Verification items for the finished model (mm, model axes). Face numbers are marked on the shaded views. A direction names the side the tool comes from. Coordinates: 2 decimals unless noted, no trailing zeros. Order: outer loops, then holes, each group sorted by start corner. A loop starts at its lowest first (then second) coordinate and runs counter-clockwise, first axis right, second up. Notation, with made-up numbers: M 36.5,59.25 L 52.5,59.25 A5 cw 52.5,66.25 Z; hole C 13.5,53 d9. An arc over 180 degrees is marked long. Answer as a JSON object with one key per item and string values. Group by question number.
(1) Material ranges on line 1 (X direction, y = -3.5, z = 15); line 2 (Z direction, x = 17, y = -8); line 3 (X direction, y = -89, z = 162), recorded low to high.
(2) Cross-section at A-A (x = 3.5). Enter the section's corners in (y, z).
(3) Access from +Z, -Z, +X, -X, +Y, -Y to the whole of each face (thin tool, end or side, straight path). Record for the marked faces 1, 2, 3, 4 and 5.
(4) Mould release check, pull along Y, two halves, no side actions. Record for the marked faces 6, 7 and 8: released by +Y, released by -Y, zero draft, split by the parting line, or undercut.
(5) Gauge pin test, flat ends, axial feed: pin 1 Ø2 at (x, z) = (-37.5, 45) entering from +Y; pin 2 Ø3 at (x, z) = (-17.5, 98) entering from +Y; pin 3 Ø5 at (x, z) = (-9.5, 44) entering from -Y. Record the tip position at first contact, or that the pin passes through.
(6) Cross-section at B-B (y = -99). Enter the section's corners in (x, z).
from build123d import *

# Parameters (mm, degrees)
ESQUISSE1_W                         = 50
ESQUISSE1_H                         = 70
ESQUISSE1_R                         = 2
ESQUISSE1_R_2                       = 20
BOSS_EXTRU_1_DEPTH                  = 10
BOSS_EXTRU_2_REACH                  = 57.317
ESQUISSE13_R                        = 21.5
ESQUISSE13_R_2                      = 20
BOSS_EXTRU_2_DIRECTION_2_DEPTH      = 90
ESQUISSE19_R                        = 21.5
ESQUISSE19_R_2                      = 20
R_VOLUTION5_ANGLE                   = 70
ESQUISSE23_R                        = 21.5
ESQUISSE23_R_2                      = 20
BOSS_EXTRU_3_DEPTH                  = 70
ESQUISSE24_W                        = 23
ESQUISSE24_H                        = 16.3
ENL_V_MAT_EXTRU_1_DEPTH             = 10
BOSS_EXTRU_4_DEPTH                  = 13
BOSS_EXTRU_4_DIRECTION_2_REACH      = 242.506
BOSS_EXTRU_4_DIRECTION_2_END_RADIUS = 21.5
ESQUISSE28_W                        = 4
ESQUISSE28_H                        = 4
BOSS_EXTRU_5_DEPTH                  = 23


with BuildPart() as part:
    # Esquisse1 → Boss.-Extru.1 (new body)
    with BuildSketch(Plane.XY):
        with Locations((-5.186655458, -0.726415094)):
            Rectangle(ESQUISSE1_W, ESQUISSE1_H)
        with Locations((-5.186655458, 25.273584906)):
            Circle(ESQUISSE1_R, mode=Mode.SUBTRACT)
        with Locations((-5.186655458, -30.726415094)):
            Circle(ESQUISSE1_R, mode=Mode.SUBTRACT)
        with Locations((-5.186655458, -0.726415094)):
            Circle(ESQUISSE1_R_2, mode=Mode.SUBTRACT)
    extrude(amount=BOSS_EXTRU_1_DEPTH)

    # Boss.-Extru.2: up to this plane
    boss_extru_2_end = Plane(origin=(0, 0, 10), z_dir=(0, 0, 1))
    # Esquisse13 → Boss.-Extru.2 (add, up to the surface)
    with BuildSketch(Plane(origin=(0, -7.393134718, 20.312470696), x_dir=(1, 0, 0), z_dir=(0, -0.34202014332566283, 0.9396926207859106)), mode=Mode.PRIVATE) as boss_extru_2_sk1:
        with Locations(Location((-5.554517745, 2.737594529, 0), (0, 0, 270))):
            Circle(ESQUISSE13_R)
        with Locations(Location((-5.554517745, 2.737594529, 0), (0, 0, 29.306498897))):
            Circle(ESQUISSE13_R_2, mode=Mode.SUBTRACT)
    boss_extru_2_tool1 = split(extrude(boss_extru_2_sk1.sketch, amount=-BOSS_EXTRU_2_REACH, mode=Mode.PRIVATE), bisect_by=boss_extru_2_end, keep=Keep.BOTH, mode=Mode.PRIVATE)
    add(boss_extru_2_tool1.solids().sort_by_distance((-5.554518, 14.811316, 28.39423))[0])

    # Esquisse13 → Boss.-Extru.2 direction 2 (add)
    with BuildSketch(Plane(origin=(0, -7.393134718, 20.312470696), x_dir=(1, 0, 0), z_dir=(0, -0.34202014332566283, 0.9396926207859106))):
        with Locations(Location((-5.554517745, 2.737594529, 0), (0, 0, 270))):
            Circle(ESQUISSE13_R)
        with Locations(Location((-5.554517745, 2.737594529, 0), (0, 0, 29.306498897))):
            Circle(ESQUISSE13_R_2, mode=Mode.SUBTRACT)
    extrude(amount=BOSS_EXTRU_2_DIRECTION_2_DEPTH)

    # Esquisse19 → Révolution5 (revolve)
    with BuildSketch(Plane(origin=(0, -38.174947617, 104.884806567), x_dir=(1, 0, 0), z_dir=(0, -0.34202014332566294, 0.9396926207859106))):
        with Locations(Location((-5.554517745, 2.737594529, 0), (0, 0, 90))):
            Circle(ESQUISSE19_R)
        with Locations(Location((-5.554517745, 2.737594529, 0), (0, 0, 90))):
            Circle(ESQUISSE19_R_2, mode=Mode.SUBTRACT)
    revolve(axis=Axis((-5.554579986, -94.784211414, 84.280719561), (1, 0, 0)), revolution_arc=R_VOLUTION5_ANGLE)

    # Esquisse23 → Boss.-Extru.3 (add)
    with BuildSketch(Plane.XZ.offset(94.784211414)):
        with Locations(Location((-5.554579986, 147.260634339, 0), (0, 0, 270))):
            Circle(ESQUISSE23_R)
        with Locations(Location((-5.554579986, 147.260634339, 0), (0, 0, 270.000178307))):
            Circle(ESQUISSE23_R_2, mode=Mode.SUBTRACT)
    extrude(amount=BOSS_EXTRU_3_DEPTH)

    # Esquisse24 → Enlèv. mat.-Extru.1 (cut)
    with BuildSketch(Plane.ZY.offset(27.186655458)):
        with Locations((46.360115203, -11.15)):
            Rectangle(ESQUISSE24_W, ESQUISSE24_H)
    extrude(amount=-ENL_V_MAT_EXTRU_1_DEPTH, mode=Mode.SUBTRACT)



with BuildPart() as body_2:
    # Esquisse27 → Boss.-Extru.4 (new body)
    with BuildSketch(Plane.ZY.offset(27.186655458)):
        Polygon((60.860115203, 0), (34.860115203, 0), (34.860115203, -3), (57.860115203, -3), (57.860115203, -19.3), (34.860115203, -19.3), (34.860115203, -22.3), (60.860115203, -22.3), align=None)
    extrude(amount=BOSS_EXTRU_4_DEPTH)

    # Boss.-Extru.4 direction 2: up to this cylinder (the profile starts outside it)
    boss_extru_4_direction_2_end = Plane(origin=(-5.554517745, -12.849515831, 43.307945529), z_dir=(0, 0.34202014332566283, -0.9396926207859105)) * Cylinder(BOSS_EXTRU_4_DIRECTION_2_END_RADIUS, 529.012, mode=Mode.PRIVATE)
    # Esquisse27 → Boss.-Extru.4 direction 2 (add, up to the surface)
    with BuildSketch(Plane.ZY.offset(27.186655458), mode=Mode.PRIVATE) as boss_extru_4_direction_2_sk1:
        Polygon((60.860115203, 0), (34.860115203, 0), (34.860115203, -3), (57.860115203, -3), (57.860115203, -19.3), (34.860115203, -19.3), (34.860115203, -22.3), (60.860115203, -22.3), align=None)
    boss_extru_4_direction_2_tool1 = extrude(boss_extru_4_direction_2_sk1.sketch, amount=-BOSS_EXTRU_4_DIRECTION_2_REACH, mode=Mode.PRIVATE) - boss_extru_4_direction_2_end
    add(boss_extru_4_direction_2_tool1.solids().sort_by_distance((-27.186655, -0.342533, 47.860115))[0])


with BuildPart() as part_1:
    add(part.part)

    add(body_2.part)  # Boss.-Extru.5 merges body 2
    # Esquisse28 → Boss.-Extru.5 (add)
    with BuildSketch(Plane(origin=(0, 0, 34.860115203), x_dir=(-1, 0, 0), z_dir=(0, 0, -1))):
        with Locations((31.138517686, -5)):
            Rectangle(ESQUISSE28_W, ESQUISSE28_H)
        with Locations((36.938517686, -5)):
            Rectangle(ESQUISSE28_W, ESQUISSE28_H)
        with Locations((31.138517686, -17.3)):
            Rectangle(ESQUISSE28_W, ESQUISSE28_H)
        with Locations((36.938517686, -17.3)):
            Rectangle(ESQUISSE28_W, ESQUISSE28_H)
    extrude(amount=-BOSS_EXTRU_5_DEPTH)


solid = part_1.part
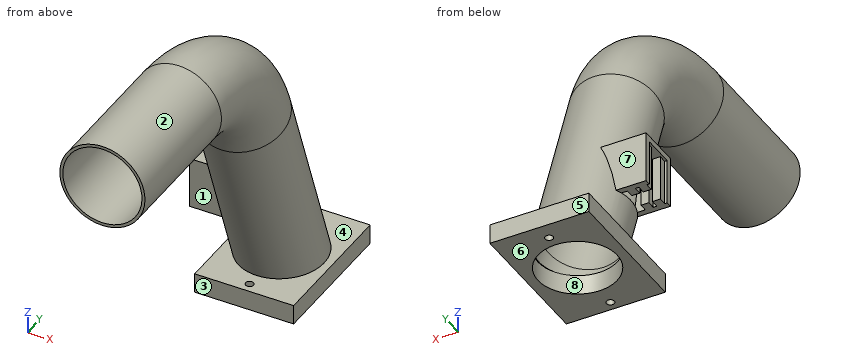
Taken from the geometry:
{
 "1": {"line 1": "x = -27.04 to -25.53, 14.43 to 15.93", "line 2": "z = 0 to 10", "line 3": "x = -21 to -18.83, 7.73 to 9.89"},
 "2": {"outline": "M -164.78,127.76 L -94.78,127.76 A43.48 cw -53.93,99.15 L -21.48,10 L -35.73,10 L -35.73,0 L -18.74,0 L -18.74,10 L -19.7,10 L -52.36,99.72 A45.15 ccw -94.78,129.43 L -164.78,129.43 Z; M -164.78,165.09 L -94.78,165.09 A80.81 cw -18.84,111.92 L 18.25,10 L 17.29,10 L 17.29,0 L 34.27,0 L 34.27,10 L 20.03,10 L -17.28,112.49 A82.48 ccw -94.78,166.76 L -164.78,166.76 Z"},
 "3": {"face 1": "-X, -Y", "face 2": "-Y", "face 3": "-Z, +X, -X, -Y", "face 4": "none", "face 5": "+Z, -Z, +X, -X, +Y"},
 "4": {"face 6": "zero draft", "face 7": "released by +Y", "face 8": "undercut"},
 "5": {"pin 1": "stops at y = 0", "pin 2": "stops at y = -12.6", "pin 3": "stops at y = -36.6"},
 "6": {"outline": "C -5.55,147.26 d43; hole C -5.55,147.26 d40"}
}
